Build history of the part. All positions in model axes, mm. A direction names the side the tool comes from. Coordinates: 2 decimals unless noted, no trailing zeros. Write each loop counter-clockwise with the first axis right and the second up, starting at its lowest first coordinate (ties: lowest second). Pieces come first, ordered by that corner, then holes.
```python
from build123d import *

# Parameters (mm, degrees)
PRISM004_DEPTH          = 5
PRISM003_DEPTH          = 5
PRISM002_DEPTH          = 5
PRISM001_DEPTH          = 5
CYLINDER016_R           = 1.7
CYLINDER016_DEPTH       = 10
CYLINDER015_R           = 1.7
CYLINDER015_DEPTH       = 10
CYLINDER014_R           = 1.7
CYLINDER014_DEPTH       = 10
CYLINDER013_R           = 1.7
CYLINDER013_DEPTH       = 10
CYLINDER012_R           = 1.7
CYLINDER012_DEPTH       = 10
CYLINDER011_R           = 1.7
CYLINDER011_DEPTH       = 10
CYLINDER010_R           = 1.7
CYLINDER010_DEPTH       = 10
CYLINDER009_R           = 1.7
CYLINDER009_DEPTH       = 10
CYLINDER008_R           = 1.7
CYLINDER008_DEPTH       = 10
CYLINDER007_R           = 1.7
CYLINDER007_DEPTH       = 10
CYLINDER006_R           = 1.7
CYLINDER006_DEPTH       = 10
CYLINDER005_R           = 1.7
CYLINDER005_DEPTH       = 10
PRISM_DEPTH             = 6.5
PRISM_PITCH_ANGLE       = 90
CYLINDER004_R           = 7.5
CYLINDER004_DEPTH       = 25
CYLINDER004_PITCH_ANGLE = 90
CYLINDER003_R           = 7.5
CYLINDER003_DEPTH       = 25
CYLINDER003_PITCH_ANGLE = 90
CYLINDER002_R           = 5
CYLINDER002_DEPTH       = 36
CYLINDER002_PITCH_ANGLE = 90
CYLINDER001_R           = 5
CYLINDER001_DEPTH       = 36
CYLINDER001_PITCH_ANGLE = 90
CYLINDER_R              = 5
CYLINDER_DEPTH          = 36
CYLINDER_PITCH_ANGLE    = 90
BOX_W                   = 36
BOX_H                   = 100
BOX_DEPTH               = 10


with BuildPart() as prisma004:
    # Prism004 → Prism004 (new body)
    with BuildSketch(Plane(origin=(18, 96, 5), x_dir=(1, 0, 0), z_dir=(0, 0, 1))):
        Polygon((3.1, 0), (1.55, 2.684679), (-1.55, 2.684679), (-3.1, 0), (-1.55, -2.684679), (1.55, -2.684679), align=None)
    extrude(amount=PRISM004_DEPTH)


with BuildPart() as prisma003:
    # Prism003 → Prism003 (new body)
    with BuildSketch(Plane(origin=(18, 67.5, 5), x_dir=(1, 0, 0), z_dir=(0, 0, 1))):
        Polygon((3.1, 0), (1.55, 2.684679), (-1.55, 2.684679), (-3.1, 0), (-1.55, -2.684679), (1.55, -2.684679), align=None)
    extrude(amount=PRISM003_DEPTH)


with BuildPart() as prisma002:
    # Prism002 → Prism002 (new body)
    with BuildSketch(Plane(origin=(18, 32.5, 5), x_dir=(1, 0, 0), z_dir=(0, 0, 1))):
        Polygon((3.1, 0), (1.55, 2.684679), (-1.55, 2.684679), (-3.1, 0), (-1.55, -2.684679), (1.55, -2.684679), align=None)
    extrude(amount=PRISM002_DEPTH)


with BuildPart() as prisma001:
    # Prism001 → Prism001 (new body)
    with BuildSketch(Plane(origin=(18, 4, 5), x_dir=(1, 0, 0), z_dir=(0, 0, 1))):
        Polygon((3.1, 0), (1.55, 2.684679), (-1.55, 2.684679), (-3.1, 0), (-1.55, -2.684679), (1.55, -2.684679), align=None)
    extrude(amount=PRISM001_DEPTH)


with BuildPart() as cilindro016:
    # Cylinder016 → Cylinder016 (new body)
    with BuildSketch(Plane(origin=(18, 96, 0), x_dir=(1, 0, 0), z_dir=(0, 0, 1))):
        Circle(CYLINDER016_R)
    extrude(amount=CYLINDER016_DEPTH)


with BuildPart() as cilindro015:
    # Cylinder015 → Cylinder015 (new body)
    with BuildSketch(Plane(origin=(18, 67.5, 0), x_dir=(1, 0, 0), z_dir=(0, 0, 1))):
        Circle(CYLINDER015_R)
    extrude(amount=CYLINDER015_DEPTH)


with BuildPart() as cilindro014:
    # Cylinder014 → Cylinder014 (new body)
    with BuildSketch(Plane(origin=(18, 32.5, 0), x_dir=(1, 0, 0), z_dir=(0, 0, 1))):
        Circle(CYLINDER014_R)
    extrude(amount=CYLINDER014_DEPTH)


with BuildPart() as cilindro013:
    # Cylinder013 → Cylinder013 (new body)
    with BuildSketch(Plane(origin=(18, 4, 0), x_dir=(1, 0, 0), z_dir=(0, 0, 1))):
        Circle(CYLINDER013_R)
    extrude(amount=CYLINDER013_DEPTH)


with BuildPart() as cilindro012:
    # Cylinder012 → Cylinder012 (new body)
    with BuildSketch(Plane(origin=(30, 96, 0), x_dir=(1, 0, 0), z_dir=(0, 0, 1))):
        Circle(CYLINDER012_R)
    extrude(amount=CYLINDER012_DEPTH)


with BuildPart() as cilindro011:
    # Cylinder011 → Cylinder011 (new body)
    with BuildSketch(Plane(origin=(6, 96, 0), x_dir=(1, 0, 0), z_dir=(0, 0, 1))):
        Circle(CYLINDER011_R)
    extrude(amount=CYLINDER011_DEPTH)


with BuildPart() as cilindro010:
    # Cylinder010 → Cylinder010 (new body)
    with BuildSketch(Plane(origin=(30, 67.5, 0), x_dir=(1, 0, 0), z_dir=(0, 0, 1))):
        Circle(CYLINDER010_R)
    extrude(amount=CYLINDER010_DEPTH)


with BuildPart() as cilindro009:
    # Cylinder009 → Cylinder009 (new body)
    with BuildSketch(Plane(origin=(6, 67.5, 0), x_dir=(1, 0, 0), z_dir=(0, 0, 1))):
        Circle(CYLINDER009_R)
    extrude(amount=CYLINDER009_DEPTH)


with BuildPart() as cilindro008:
    # Cylinder008 → Cylinder008 (new body)
    with BuildSketch(Plane(origin=(30, 32.5, 0), x_dir=(1, 0, 0), z_dir=(0, 0, 1))):
        Circle(CYLINDER008_R)
    extrude(amount=CYLINDER008_DEPTH)


with BuildPart() as cilindro007:
    # Cylinder007 → Cylinder007 (new body)
    with BuildSketch(Plane(origin=(6, 32.5, 0), x_dir=(1, 0, 0), z_dir=(0, 0, 1))):
        Circle(CYLINDER007_R)
    extrude(amount=CYLINDER007_DEPTH)


with BuildPart() as cilindro006:
    # Cylinder006 → Cylinder006 (new body)
    with BuildSketch(Plane(origin=(30, 4, 0), x_dir=(1, 0, 0), z_dir=(0, 0, 1))):
        Circle(CYLINDER006_R)
    extrude(amount=CYLINDER006_DEPTH)


with BuildPart() as cilindro005:
    # Cylinder005 → Cylinder005 (new body)
    with BuildSketch(Plane(origin=(6, 4, 0), x_dir=(1, 0, 0), z_dir=(0, 0, 1))):
        Circle(CYLINDER005_R)
    extrude(amount=CYLINDER005_DEPTH)


with BuildPart() as prisma:
    # Prism → Prism (new body)
    with BuildSketch(Plane.XY):
        Polygon((8.5, 0), (4.25, 7.361216), (-4.25, 7.361216), (-8.5, 0), (-4.25, -7.361216), (4.25, -7.361216), align=None)
    extrude(amount=PRISM_DEPTH)


with BuildPart() as prisma_1:
    # Prism pitch: moved
    add(prisma.part.rotate(Axis((0, 0, 0), (0, 1, 0)), PRISM_PITCH_ANGLE))


with BuildPart() as prisma_2:
    # Prism placement: moved
    add(prisma_1.part.moved(Location((14.75, 50, 10))))


with BuildPart() as cilindro004:
    # Cylinder004 → Cylinder004 (new body)
    with BuildSketch(Plane.XY):
        Circle(CYLINDER004_R)
    extrude(amount=CYLINDER004_DEPTH)


with BuildPart() as cilindro004_1:
    # Cylinder004 pitch: moved
    add(cilindro004.part.rotate(Axis((0, 0, 0), (0, 1, 0)), CYLINDER004_PITCH_ANGLE))


with BuildPart() as cilindro004_2:
    # Cylinder004 placement: moved
    add(cilindro004_1.part.moved(Location((5.5, 85, 10))))


with BuildPart() as cilindro003:
    # Cylinder003 → Cylinder003 (new body)
    with BuildSketch(Plane.XY):
        Circle(CYLINDER003_R)
    extrude(amount=CYLINDER003_DEPTH)


with BuildPart() as cilindro003_1:
    # Cylinder003 pitch: moved
    add(cilindro003.part.rotate(Axis((0, 0, 0), (0, 1, 0)), CYLINDER003_PITCH_ANGLE))


with BuildPart() as cilindro003_2:
    # Cylinder003 placement: moved
    add(cilindro003_1.part.moved(Location((5.5, 15, 10))))


with BuildPart() as cilindro002:
    # Cylinder002 → Cylinder002 (new body)
    with BuildSketch(Plane.XY):
        Circle(CYLINDER002_R)
    extrude(amount=CYLINDER002_DEPTH)


with BuildPart() as cilindro002_1:
    # Cylinder002 pitch: moved
    add(cilindro002.part.rotate(Axis((0, 0, 0), (0, 1, 0)), CYLINDER002_PITCH_ANGLE))


with BuildPart() as cilindro002_2:
    # Cylinder002 placement: moved
    add(cilindro002_1.part.moved(Location((0, 85, 10))))


with BuildPart() as cilindro001:
    # Cylinder001 → Cylinder001 (new body)
    with BuildSketch(Plane.XY):
        Circle(CYLINDER001_R)
    extrude(amount=CYLINDER001_DEPTH)


with BuildPart() as cilindro001_1:
    # Cylinder001 pitch: moved
    add(cilindro001.part.rotate(Axis((0, 0, 0), (0, 1, 0)), CYLINDER001_PITCH_ANGLE))


with BuildPart() as cilindro001_2:
    # Cylinder001 placement: moved
    add(cilindro001_1.part.moved(Location((0, 50, 10))))


with BuildPart() as cilindro:
    # Cylinder → Cylinder (new body)
    with BuildSketch(Plane.XY):
        Circle(CYLINDER_R)
    extrude(amount=CYLINDER_DEPTH)


with BuildPart() as cilindro_1:
    # Cylinder pitch: moved
    add(cilindro.part.rotate(Axis((0, 0, 0), (0, 1, 0)), CYLINDER_PITCH_ANGLE))


with BuildPart() as cilindro_2:
    # Cylinder placement: moved
    add(cilindro_1.part.moved(Location((0, 15, 10))))


with BuildPart() as cut021:
    # Box → Box (new body)
    with BuildSketch(Plane.XY):
        with Locations((18, 50)):
            Rectangle(BOX_W, BOX_H)
    extrude(amount=BOX_DEPTH)

    # Cut: cut Cilindro
    add(cilindro_2.part, mode=Mode.SUBTRACT)

    # Cut001: cut Cilindro001
    add(cilindro001_2.part, mode=Mode.SUBTRACT)

    # Cut002: cut Cilindro002
    add(cilindro002_2.part, mode=Mode.SUBTRACT)

    # Cut003: cut Cilindro003
    add(cilindro003_2.part, mode=Mode.SUBTRACT)

    # Cut004: cut Cilindro004
    add(cilindro004_2.part, mode=Mode.SUBTRACT)

    # Cut005: cut Prisma
    add(prisma_2.part, mode=Mode.SUBTRACT)

    # Cut006: cut Cilindro005
    add(cilindro005.part, mode=Mode.SUBTRACT)

    # Cut007: cut Cilindro006
    add(cilindro006.part, mode=Mode.SUBTRACT)

    # Cut008: cut Cilindro007
    add(cilindro007.part, mode=Mode.SUBTRACT)

    # Cut009: cut Cilindro008
    add(cilindro008.part, mode=Mode.SUBTRACT)

    # Cut010: cut Cilindro009
    add(cilindro009.part, mode=Mode.SUBTRACT)

    # Cut011: cut Cilindro010
    add(cilindro010.part, mode=Mode.SUBTRACT)

    # Cut012: cut Cilindro011
    add(cilindro011.part, mode=Mode.SUBTRACT)

    # Cut013: cut Cilindro012
    add(cilindro012.part, mode=Mode.SUBTRACT)

    # Cut014: cut Cilindro013
    add(cilindro013.part, mode=Mode.SUBTRACT)

    # Cut015: cut Cilindro014
    add(cilindro014.part, mode=Mode.SUBTRACT)

    # Cut016: cut Cilindro015
    add(cilindro015.part, mode=Mode.SUBTRACT)

    # Cut017: cut Cilindro016
    add(cilindro016.part, mode=Mode.SUBTRACT)

    # Cut018: cut Prisma001
    add(prisma001.part, mode=Mode.SUBTRACT)

    # Cut019: cut Prisma002
    add(prisma002.part, mode=Mode.SUBTRACT)

    # Cut020: cut Prisma003
    add(prisma003.part, mode=Mode.SUBTRACT)

    # Cut021: cut Prisma004
    add(prisma004.part, mode=Mode.SUBTRACT)


solid = cut021.part
```
1. Saw through at B-B on y = 47.5. List the corners of the cut face in (x, z).
Computed values:
outline: (0, 0) - (36, 0) - (36, 5.67) - (21.25, 5.67) - (21.25, 2.94) - (14.75, 2.94) - (14.75, 5.67) - (0, 5.67) - close
2. Flat gauge pin, fed straight in: pin 1 (1.6 mm diameter, centred on x = 17.5, y = 31.5, fed in from +Z). Where does the tip first touch, or does it go through?
Computed values:
pin 1: stops at z = 5
3. Saw through at C-C on z = 7.5. State how many separate pieces and enclosed holes the cut face has, plus the area to 3 significant figures.
Computed values:
separate pieces: 4
enclosed holes: 12
area: 2,180 mm2
4. Mould opens along Y. For faces 1 (the face through (17.7, 70.5, 10)), 2 (the face through (18, 100, 5)), 3 (the face through (18, 64.815, 7)) say: +Y half, -Y half, draft (parallel to the pull), parting line (faces both ways), or undercut.
Computed values:
face 1: draft
face 2: +Y half
face 3: undercut
5. 3-axis set-ups, long thin cutter, end or side, ignore diameter. For faces 4 (the face through (3, 15, 5)), 5 (the face through (15.66, 31.18, 7.46)): which of +Z, -Z, +X, -X, +Y, -Y reach the whole face in a straight line?
Computed values:
face 4: +Z, +X, -X
face 5: +Z
6. Saw through at A-A on x = 13. List the corners of the cut face in (y, z), plus the area to 3 significant figures.
Computed values:
outline: (0, 0) - (100, 0) - (100, 10) - (92.5, 10) arc R7.5 cw to (77.5, 10) - (55, 10) arc R5 cw to (45, 10) - (22.5, 10) arc R7.5 cw to (7.5, 10) - (0, 10) - close
area: 784 mm2
7. Saw through at D-D on y = 21.5. List the corners of the cut face in (x, z).
Computed values:
outline: (0, 0) - (36, 0) - (36, 10) - (30.5, 10) - (30.5, 6.26) - (5.5, 6.26) - (5.5, 10) - (0, 10) - close
8. Probe line 1 along X through (y, z) = (67.5, 4); line 2 along X through (y, z) = (96, 5.25); line 3 along Y through (x, z) = (18, 2.45). List the from-to ranges inside material, lowest first.
Computed values:
line 1: x = 0 to 4.3, 7.7 to 16.3, 19.7 to 28.3, 31.7 to 36
line 2: x = 0 to 4.3, 7.7 to 14.9, 21.1 to 28.3, 31.7 to 36
line 3: y = 0 to 2.3, 5.7 to 30.8, 34.2 to 48.35, 51.65 to 65.8, 69.2 to 94.3, 97.7 to 100
